from build123d import *

# Parameters (mm, degrees)
SKETCH1_R                     = 17
BOSS_EXTRUDE1_DEPTH           = 24.88
SKETCH2_W                     = 14
SKETCH2_H                     = 44
BOSS_EXTRUDE2_DEPTH           = 11
CSK_FOR_M5_SFHCS1_D           = 5.3
CSK_FOR_M5_SFHCS1_CSINK_D     = 11.2
CSK_FOR_M5_SFHCS1_CSINK_ANGLE = 90


with BuildPart() as part:
    # Sketch1 → Boss-Extrude1 (new body)
    with BuildSketch(Plane(origin=(0, 0, 0), x_dir=(1, 0, 0), z_dir=(0, 1, 0))):
        Circle(SKETCH1_R)
    extrude(amount=BOSS_EXTRUDE1_DEPTH)

    # Sketch2 → Boss-Extrude2 (add)
    with BuildSketch(Plane(origin=(0, 24.88, 0), x_dir=(1, 0, 0), z_dir=(0, 1, 0))):
        Rectangle(SKETCH2_W, SKETCH2_H)
    extrude(amount=-BOSS_EXTRUDE2_DEPTH)

    # CSK for M5 SFHCS1 (through all)
    with Locations(Plane(origin=(0, 24.88, 0), x_dir=(1, 0, 0), z_dir=(0, 1, 0))):
        with Locations((0, 0)):
            CounterSinkHole(CSK_FOR_M5_SFHCS1_D / 2, CSK_FOR_M5_SFHCS1_CSINK_D / 2, counter_sink_angle=CSK_FOR_M5_SFHCS1_CSINK_ANGLE)


solid = part.part
CAD build for the part. Positions are in the model's coordinates, mm. A direction names the side the tool comes from. Round coordinates to 2 decimals unless told otherwise and drop trailing zeros. Loops run counter-clockwise (first coordinate to the right, second up) from the corner with the lowest first, then second, coordinate; pieces in that order, holes last.
(1) Cut at A-A (z = 0). Give the cut face in (x, y).
(2) Cut at B-B (x = 0). Give the cut face in (y, z).
(3) Cut at C-C (y = 19). Give the cut face in (x, z), plus the area to 3 significant figures.
(4) Wall check: line 1 along Z through (x, y) = (0, 8); line 2 along Z through (x, y) = (0, 14); line 3 along Y through (x, z) = (5, 2.5). Give the ranges that are in metal, low to high.
(5) Which spindle directions (+Z, -Z, +X, -X, +Y, -Y) get a long thin tool onto all of the face, cutting with end or side? Do faces 1 (the flat face through (7, 19, 19)), 2 (the cylindrical face through (16.215, 12.266, -5.106)), 3 (the flat face through (-7, 19, 19)), 4 (the flat face through (7, 19, -19)). Say none if no direction does.
(6) Two-plate mould, pull along X, no slides. Class faces 5 (the cylindrical face through (-2.45, 10.81, 1.01)), 6 (the flat face through (-7, 19, -19)), 7 (the flat face through (0, 13.88, -20)), 8 (the conical face through (-2.66, 22.07, -0.84)): +X half, -X half, draft (parallel to the pull), parting line (faces both ways), or undercut.
(7) Cut at D-D (x = -8). Give the cut face in (y, z), plus the area to 3 significant figures.
(8) Drop flat-ended pins along their axis: pin 1 (3.5 mm diameter, centred on y = 20, z = -18, fed in from +X); pin 2 (10 mm diameter, centred on y = 19, z = 8, fed in from -X); pin 3 (2 mm diameter, centred on x = 0, z = 19.5, fed in from -Y); pin 4 (5 mm diameter, centred on x = 1.5, z = -17.5, fed in from -Y). Give the stop position or say it passes through.
Findings below:
1. outline: (-17, 0) - (-2.65, 0) - (-2.65, 21.93) - (-5.6, 24.88) - (-17, 24.88) - close; (2.65, 0) - (17, 0) - (17, 24.88) - (5.6, 24.88) - (2.65, 21.93) - close
2. outline: (0, -17) - (13.88, -17) - (13.88, -22) - (24.88, -22) - (24.88, -5.6) - (21.93, -2.65) - (0, -2.65) - close; (0, 2.65) - (21.93, 2.65) - (24.88, 5.6) - (24.88, 22) - (13.88, 22) - (13.88, 17) - (0, 17) - close
3. outline: (-7, -22) - (7, -22) - (7, -15.49) arc R17 ccw to (7, 15.49) - (7, 22) - (-7, 22) - (-7, 15.49) arc R17 ccw to (-7, -15.49) - close; hole circle Ø5.3 at (0, 0)
3. area: 1,040 mm2
4. line 1: z = -17 to -2.65, 2.65 to 17
4. line 2: z = -22 to -2.65, 2.65 to 22
4. line 3: y = 0 to 24.87
5. face 1: +Z, +X, +Y, -Y
5. face 2: -Y
5. face 3: +Z, -X, +Y, -Y
5. face 4: -Z, +X, +Y, -Y
6. face 5: undercut
6. face 6: -X half
6. face 7: draft
6. face 8: undercut
7. outline: (0, -15) - (24.88, -15) - (24.88, 15) - (0, 15) - close
7. area: 746 mm2
8. pin 1: stops at x = 7
8. pin 2: stops at x = -16.73
8. pin 3: stops at y = 13.88
8. pin 4: stops at y = 0
